```python
from build123d import *

# Parameters (mm, degrees)
F0_W         = 152.4
F0_H         = 76.2
F1_DEPTH     = 12.7
F2_R         = 12.7
F3_DEPTH     = 12.7
F4_R         = 12.7
F5_DEPTH     = 12.7
F6_R         = 12.7
F7_DEPTH     = 12.7
F8_W         = 25.4
F8_H         = 50.8
F11_W        = 22.735084407
F11_H        = 25.6498381495
F13_R        = 5.08
F14_T1_DEPTH = 178.5282991577
F14_T3_DEPTH = 102.3282991577


# Not quite as in the source:
# - a fillet or chamfer that OpenCascade refuses, or shapes differently, is made with other operations: its cross-section is extruded or revolved along the edge and cut away or added


with BuildPart() as f1:
    # F0 (on Top) → F1 (new body)
    with BuildSketch(Plane.XY):
        Rectangle(F0_W, F0_H)
    extrude(amount=F1_DEPTH)

    # F2 (on face) → F3 (cut)
    with BuildSketch(Plane.XY.offset(12.7)):
        with Locations((57.0033815651, -19.0182915657)):
            Circle(F2_R)
    extrude(amount=-F3_DEPTH, mode=Mode.SUBTRACT)

    # F4 (on Top) → F5 (cut)
    with BuildSketch(Plane.XY):
        with Locations((-55.634457748, -18.9344183354)):
            Circle(F4_R)
    extrude(amount=F5_DEPTH, mode=Mode.SUBTRACT)

    # F6 (on Top) → F7 (cut)
    with BuildSketch(Plane.XY):
        with Locations((-56.6692140824, 22.2065947787)):
            Circle(F6_R)
        with Locations((58.9656175097, 22.9479158466)):
            Circle(F6_R)
    extrude(amount=F7_DEPTH, mode=Mode.SUBTRACT)

    # F8 (on Front) → F9 (revolve)
    with BuildSketch(Plane.XZ):
        with Locations((12.7, 38.1)):
            Rectangle(F8_W, F8_H)
    revolve(axis=Axis((0, 0, 38.1), (0, 0, 1)))

    # F11 (on Front) → F12 (revolve, cut)
    with BuildSketch(Plane.XZ):
        with Locations((-23.9009843208, 39.7863946855)):
            Rectangle(F11_W, F11_H)
    revolve(axis=Axis((0, 0, 31.6979512572), (0, 0, 1)), mode=Mode.SUBTRACT)

    # F13
    f13_edges = [f1.edges().sort_by_distance(p)[0] for p in [
        (-25.4, 0, 63.5),
        (-25.4, 0, 26.961476),
        (-25.4, 0, 12.7),
    ]]
    fillet(f13_edges, radius=F13_R)

    # F14: chamfer of 5.08 on 4 edges, made by hand

    # F14_s2 → F14_t1 (cut)
    with BuildSketch(Plane.YZ.offset(-89.2641495789)):
        Polygon((-33.02, 12.7), (-38.1, 7.62), (-38.1, 12.7), align=None)
        Polygon((33.02, 12.7), (38.1, 7.62), (38.1, 12.7), align=None)
    extrude(amount=F14_T1_DEPTH, mode=Mode.SUBTRACT)

    # F14_s4 → F14_t3 (cut)
    with BuildSketch(Plane.XZ.offset(-51.1641495789)):
        Polygon((-71.12, 12.7), (-76.2, 7.62), (-76.2, 12.7), align=None)
        Polygon((71.12, 12.7), (76.2, 7.62), (76.2, 12.7), align=None)
    extrude(amount=F14_T3_DEPTH, mode=Mode.SUBTRACT)


solid = f1.part
```
Input: part model. Units: mm. Frame: model coordinates. A direction names the side the tool comes from. Coordinates: 2 decimals unless noted, no trailing zeros. Write each loop counter-clockwise with the first axis right and the second up, starting at its lowest first coordinate (ties: lowest second). Pieces come first, ordered by that corner, then holes. Notation, with made-up numbers: (-5.5, -4) -> (11.5, -4) arc R30 cw to (11.5, 19) -> close; hole circle Ø1 at (34.25, 19). An arc over 180 degrees is marked (long way). Write each question's results on one line, items separated by ' | '.
Item 1: Material intervals for probe 1 along Y at (x, z) = (52, 9); probe 2 along Y at (x, z) = (-53.5, 3); probe 3 along Z at (x, y) = (-41, 28.5), sorted ascending.
Conclusion:
probe 1: y = -36.72 to -30.69, -7.35 to 12.33, 33.57 to 36.72 | probe 2: y = -38.1 to -31.45, -6.42 to 9.91, 34.5 to 38.1 | probe 3: z = 0 to 12.7
Item 2: Section query C-C on z = 48.5. Return loops of the section in (x, y).
Conclusion:
outline: circle Ø25.07 at (0, 0)
Item 3: Set-up query: faces 4 (the flat face through (70, 31, 12.7)), 5 (the cylindrical face through (-5.506, -24.796, 55.556)), 6 (the cylindrical face through (2.717, 12.235, 39.966)). Return all of +Z, -Z, +X, -X, +Y, -Y with unobstructed straight access to the full face (end or side cutting, diameter ignored); none if empty.
Conclusion:
face 4: +Z, +X, +Y, -Y | face 5: +Z | face 6: none
Item 4: Pin query (flat end, axial travel): pin 1 Ø23 at (x, y) = (58.97, 22.95) entering from -Z; pin 2 Ø8 at (y, z) = (17, 14) entering from -X; pin 3 Ø1.5 at (x, z) = (-18.5, 8.5) entering from +Y; pin 4 Ø4 at (x, y) = (42, -26) entering from +Z. Return the tip coordinate at first contact, or that it passes through.
Conclusion:
pin 1: passes through | pin 2: stops at x = -73.82 | pin 3: stops at y = 37.97 | pin 4: stops at z = 12.7
Item 5: Section query D-D on x = 35. Return loops of the section in (y, z), plus the area to 3 significant figures.
Conclusion:
outline: (-38.1, 0) -> (38.1, 0) -> (38.1, 7.62) -> (33.02, 12.7) -> (-33.02, 12.7) -> (-38.1, 7.62) -> close | area: 942 mm^2
Item 6: Section query A-A on x = 0. Return loops of the section in (y, z), plus the area to 3 significant figures.
Conclusion:
outline: (-38.1, 0) -> (38.1, 0) -> (38.1, 7.62) -> (33.02, 12.7) -> (30.48, 12.7) arc R5.08 cw to (25.4, 17.78) -> (25.4, 21.88) arc R5.08 ccw to (20.32, 26.96) -> (12.53, 26.96) -> (12.53, 52.61) -> (25.4, 52.61) -> (25.4, 58.42) arc R5.08 ccw to (20.32, 63.5) -> (-20.32, 63.5) arc R5.08 ccw to (-25.4, 58.42) -> (-25.4, 52.61) -> (-12.53, 52.61) -> (-12.53, 26.96) -> (-20.32, 26.96) arc R5.08 ccw to (-25.4, 21.88) -> (-25.4, 17.78) arc R5.08 cw to (-30.48, 12.7) -> (-33.02, 12.7) -> (-38.1, 7.62) -> close | area: 2,850 mm^2
Item 7: Section query B-B on y = 0. Return loops of the section in (x, z).
Conclusion:
outline: (-76.2, 0) -> (76.2, 0) -> (76.2, 7.62) -> (71.12, 12.7) -> (30.48, 12.7) arc R5.08 cw to (25.4, 17.78) -> (25.4, 21.88) arc R5.08 ccw to (20.32, 26.96) -> (12.53, 26.96) -> (12.53, 52.61) -> (25.4, 52.61) -> (25.4, 58.42) arc R5.08 ccw to (20.32, 63.5) -> (-20.32, 63.5) arc R5.08 ccw to (-25.4, 58.42) -> (-25.4, 52.61) -> (-12.53, 52.61) -> (-12.53, 26.96) -> (-20.32, 26.96) arc R5.08 ccw to (-25.4, 21.88) -> (-25.4, 17.78) arc R5.08 cw to (-30.48, 12.7) -> (-71.12, 12.7) -> (-76.2, 7.62) -> close
Item 8: Mould query, pull axis Y, two halves, no side actions, for faces 1 (the flat face through (-1.07, -35.52, 10.2)), 2 (the flat face through (9, 9, 26.961)), 3 (the cylindrical face through (46.93, -26.75, 6.44)). Classes: +Y half, -Y half, draft (parallel to the pull), parting line (faces both ways), or undercut.
Conclusion:
face 1: -Y half | face 2: draft | face 3: undercut
